```python
from build123d import *

# Parameters (mm, degrees)
SKETCH1_W            = 150.1
SKETCH1_H            = 55.1
SKETCH1_R            = 1.5
BOSS_EXTRUDE1_DEPTH  = 1.7
SKETCH2_W            = 40.8
SKETCH2_H            = 2.5
BOSS_EXTRUDE2_DEPTH  = 2.4
SKETCH3_W            = 98
SKETCH3_H            = 60
SKETCH3_R            = 1.5
BOSS_EXTRUDE3_DEPTH  = 1.6
SKETCH4_W            = 98
SKETCH4_H            = 39.8
BOSS_EXTRUDE4_DEPTH  = 10
SKETCH5_W            = 75.5
SKETCH5_H            = 25.6
CUT_EXTRUDE1_DEPTH   = 0.8
SKETCH6_R            = 6
BOSS_EXTRUDE5_DEPTH  = 9.5
SKETCH7_W            = 6
SKETCH7_H            = 6
BOSS_EXTRUDE6_DEPTH  = 3
SKETCH8_R            = 1.75
BOSS_EXTRUDE7_DEPTH  = 1.7
SKETCH9_W            = 14.7
SKETCH9_H            = 12
BOSS_EXTRUDE8_DEPTH  = 6.9
SKETCH10_R           = 3.35
BOSS_EXTRUDE9_DEPTH  = 6.9
SKETCH11_R           = 7.4
BOSS_EXTRUDE10_DEPTH = 15
SKETCH12_W           = 26.5
SKETCH12_H           = 26.5
BOSS_EXTRUDE11_DEPTH = 2.8
SKETCH13_R           = 4.6
BOSS_EXTRUDE12_DEPTH = 7.6
SKETCH14_W           = 43.1
SKETCH14_H           = 8.6
BOSS_EXTRUDE13_DEPTH = 18


with BuildPart() as part:
    # Sketch1 → Boss-Extrude1 (new body)
    with BuildSketch(Plane(origin=(0, 0, 0), x_dir=(1, 0, 0), z_dir=(0, 1, 0))):
        Rectangle(SKETCH1_W, SKETCH1_H)
        with Locations(Location((-72.35, 24.85, 0), (0, 0, 270))):
            Circle(SKETCH1_R, mode=Mode.SUBTRACT)
        with Locations(Location((-72.35, -24.85, 0), (0, 0, 270))):
            Circle(SKETCH1_R, mode=Mode.SUBTRACT)
        with Locations(Location((72.35, 24.85, 0), (0, 0, 270))):
            Circle(SKETCH1_R, mode=Mode.SUBTRACT)
        with Locations(Location((72.35, -24.85, 0), (0, 0, 270))):
            Circle(SKETCH1_R, mode=Mode.SUBTRACT)
    extrude(amount=BOSS_EXTRUDE1_DEPTH)

    # Sketch2 → Boss-Extrude2 (add)
    with BuildSketch(Plane(origin=(0, 1.7, 0), x_dir=(1, 0, 0), z_dir=(0, 1, 0))):
        with Locations((-32.85, 21.9)):
            Rectangle(SKETCH2_W, SKETCH2_H)
    extrude(amount=BOSS_EXTRUDE2_DEPTH)

    # Sketch3 → Boss-Extrude3 (add)
    with BuildSketch(Plane(origin=(0, 4.1, 0), x_dir=(1, 0, 0), z_dir=(0, 1, 0))):
        with Locations((-12.55, -5.9)):
            Rectangle(SKETCH3_W, SKETCH3_H)
        with Locations(Location((-59.05, 21.6, 0), (0, 0, 270))):
            Circle(SKETCH3_R, mode=Mode.SUBTRACT)
        with Locations(Location((33.95, 21.6, 0), (0, 0, 270))):
            Circle(SKETCH3_R, mode=Mode.SUBTRACT)
        with Locations(Location((33.95, -33.4, 0), (0, 0, 270))):
            Circle(SKETCH3_R, mode=Mode.SUBTRACT)
        with Locations(Location((-59.05, -33.4, 0), (0, 0, 270))):
            Circle(SKETCH3_R, mode=Mode.SUBTRACT)
    extrude(amount=BOSS_EXTRUDE3_DEPTH)

    # Sketch4 → Boss-Extrude4 (add)
    with BuildSketch(Plane(origin=(0, 5.7, 0), x_dir=(1, 0, 0), z_dir=(0, 1, 0))):
        with Locations((-12.55, -5.9)):
            Rectangle(SKETCH4_W, SKETCH4_H)
    extrude(amount=BOSS_EXTRUDE4_DEPTH)

    # Sketch5 → Cut-Extrude1 (cut)
    with BuildSketch(Plane(origin=(0, 15.7, 0), x_dir=(1, 0, 0), z_dir=(0, 1, 0))):
        with Locations((-12.1, -6)):
            Rectangle(SKETCH5_W, SKETCH5_H)
    extrude(amount=-CUT_EXTRUDE1_DEPTH, mode=Mode.SUBTRACT)

    # Sketch6 → Boss-Extrude5 (add)
    with BuildSketch(Plane(origin=(0, 1.7, 0), x_dir=(1, 0, 0), z_dir=(0, 1, 0))):
        with Locations(Location((61.15, 16.95, 0), (0, 0, 90))):
            Circle(SKETCH6_R)
    extrude(amount=BOSS_EXTRUDE5_DEPTH)

    # Sketch7 → Boss-Extrude6 (add)
    with BuildSketch(Plane(origin=(0, 1.7, 0), x_dir=(1, 0, 0), z_dir=(0, 1, 0))):
        with Locations((61.85, -19.35)):
            Rectangle(SKETCH7_W, SKETCH7_H)
    extrude(amount=BOSS_EXTRUDE6_DEPTH)

    # Sketch8 → Boss-Extrude7 (add)
    with BuildSketch(Plane(origin=(0, 4.7, 0), x_dir=(1, 0, 0), z_dir=(0, 1, 0))):
        with Locations(Location((61.85, -19.35, 0), (0, 0, 270))):
            Circle(SKETCH8_R)
    extrude(amount=BOSS_EXTRUDE7_DEPTH)

    # Sketch9 → Boss-Extrude8 (add)
    with BuildSketch(Plane(origin=(0, 1.7, 0), x_dir=(1, 0, 0), z_dir=(0, 1, 0))):
        with Locations((61.7, -2.35)):
            Rectangle(SKETCH9_W, SKETCH9_H)
    extrude(amount=BOSS_EXTRUDE8_DEPTH)

    # Sketch10 → Boss-Extrude9 (add)
    with BuildSketch(Plane(origin=(0, 8.6, 0), x_dir=(1, 0, 0), z_dir=(0, 1, 0))):
        with Locations(Location((61.7, -2.7, 0), (0, 0, 90))):
            Circle(SKETCH10_R)
    extrude(amount=BOSS_EXTRUDE9_DEPTH)

    # Sketch11 → Boss-Extrude10 (add)
    with BuildSketch(Plane(origin=(0, 15.5, 0), x_dir=(1, 0, 0), z_dir=(0, 1, 0))):
        with Locations(Location((61.7, -2.7, 0), (0, 0, 270))):
            Circle(SKETCH11_R)
    extrude(amount=BOSS_EXTRUDE10_DEPTH)

    # Sketch12 → Boss-Extrude11 (add)
    with BuildSketch(Plane(origin=(0, 0, 0), x_dir=(-1, 0, 0), z_dir=(0, -1, 0))):
        with Locations((61.8, -6.3)):
            Rectangle(SKETCH12_W, SKETCH12_H)
    extrude(amount=BOSS_EXTRUDE11_DEPTH)

    # Sketch13 → Boss-Extrude12 (add)
    with BuildSketch(Plane.XZ):
        with Locations(Location((-62.15, -16.85, 0), (0, 0, 90))):
            Circle(SKETCH13_R)
    extrude(amount=BOSS_EXTRUDE12_DEPTH)

    # Sketch14 → Boss-Extrude13 (add)
    with BuildSketch(Plane.XZ):
        with Locations((-7.2, -0.95)):
            Rectangle(SKETCH14_W, SKETCH14_H)
    extrude(amount=BOSS_EXTRUDE13_DEPTH)


solid = part.part
```
Work out the finished part from the listing and answer in its coordinate system (mm). A direction names the side the tool comes from. Coordinates: 2 decimals unless noted, no trailing zeros. Write each loop counter-clockwise with the first axis right and the second up, starting at its lowest first coordinate (ties: lowest second). Pieces come first, ordered by that corner, then holes. Notation, with made-up numbers: (66, -3) - (88, -3) arc R6 ccw to (88, 1) - close; hole circle Ø6 at (68, 82.5). An arc over 180 degrees is marked (long way). Answer as a JSON object with one key per item and string values.
Q1. Which of the six approach directions +Z, -Z, +X, -X, +Y, -Y give full straight-line access (tool end or side, diameter ignored) to faces 1 (the flat face through (36.45, 10, 6)), 2 (the flat face through (64.85, 3, 19)), 3 (the flat face through (58.85, 3, 19)), 4 (the cylindrical face through (60.886, 6.384, -10.956))?
Results list:
{"face 1": "+Z, -Z, +Y", "face 2": "+Z, +X, +Y", "face 3": "+Z, +Y", "face 4": "+Y"}
Q2. Find section D-D (z = -16.85). Write down the section's boundary in (x, y), plus the area to 3 significant figures.
Results list:
{"outline": "(-75.05, 0) - (-66.75, 0) - (-66.75, -7.6) - (-57.55, -7.6) - (-57.55, 0) - (75.05, 0) - (75.05, 1.7) - (67.15, 1.7) - (67.15, 11.2) - (55.15, 11.2) - (55.15, 1.7) - (-75.05, 1.7) - close; (-61.55, 4.1) - (36.45, 4.1) - (36.45, 5.7) - (-61.55, 5.7) - close", "area": "596 mm^2"}
Q3. For a pull along X with two mould halves and no side action, classify faces 5 (the cylindrical face through (-57.66, -3.75, -17.85)), 6 (the flat face through (-62, -2.8, 6)), 7 (the cylindrical face through (-71.085, 0.838, -24.044)) as pulls with the +X half, pulls with the -X half, needs draft (parallel to the pull), parting line crosses it, or undercut.
Results list:
{"face 5": "parting line crosses it", "face 6": "needs draft", "face 7": "undercut"}
Q4. Given pin 1 Ø9.5 at (y, z) = (-10.5, -1) entering from -X; pin 2 Ø5 at (x, y) = (-1, 10) entering from -Z; pin 3 Ø1 at (x, z) = (61.5, 19) entering from +Y, each flat-ended and moving along its own axis, determine where each tip first touches the part or whether it passes through.
Results list:
{"pin 1": "stops at x = -28.75", "pin 2": "stops at z = -14", "pin 3": "stops at y = 6.4"}
Q5. Find section C-C (x = -34.5). Write down the section's boundary in (y, z).
Results list:
{"outline": "(0, -27.55) - (1.7, -27.55) - (1.7, -23.15) - (4.1, -23.15) - (4.1, -24.1) - (5.7, -24.1) - (5.7, -14) - (15.7, -14) - (15.7, -6.8) - (14.9, -6.8) - (14.9, 18.8) - (15.7, 18.8) - (15.7, 25.8) - (5.7, 25.8) - (5.7, 35.9) - (4.1, 35.9) - (4.1, -20.65) - (1.7, -20.65) - (1.7, 27.55) - (0, 27.55) - close"}
Q6. Consider L1, parallel to X at y = 1.15, z = -24.85; L2, parallel to Y at x = -42, z = 1; L3, parallel to Y at x = -57, z = 10.5. Determine where each line is inside the solid, lowest interval first. Write a range as from..to.
Results list:
{"L1": "x = -75.05..-73.85, -70.85..70.85, 73.85..75.05", "L2": "y = 0..1.7, 4.1..14.9", "L3": "y = -2.8..1.7, 4.1..15.7"}
Q7. Find section B-B (y = 13). Write down the section's boundary in (x, z), plus the area to 3 significant figures.
Results list:
{"outline": "(-61.55, -14) - (36.45, -14) - (36.45, 25.8) - (-61.55, 25.8) - close; circle Ø6.7 at (61.7, 2.7)", "area": "3,940 mm^2"}
Q8. Find section A-A (x = 17.5). Write down the section's boundary in (y, z), plus the area to 3 significant figures.
Results list:
{"outline": "(0, -27.55) - (1.7, -27.55) - (1.7, 27.55) - (0, 27.55) - close; (4.1, -24.1) - (5.7, -24.1) - (5.7, -14) - (15.7, -14) - (15.7, -6.8) - (14.9, -6.8) - (14.9, 18.8) - (15.7, 18.8) - (15.7, 25.8) - (5.7, 25.8) - (5.7, 35.9) - (4.1, 35.9) - close", "area": "567 mm^2"}
